from build123d import *

# Parameters (mm, degrees)
F0_W     = 14.1024803743
F0_H     = 7.6268524863
F1_DEPTH = 1
F2_W     = 9.7692511044
F2_H     = 7.6268524863
F3_DEPTH = 12.8
F5_DEPTH = 7.65
F6_R     = 2.220289971
F7_DEPTH = 5


with BuildPart() as f1:
    # F0 (on Front) → F1 (new body)
    with BuildSketch(Plane.XZ):
        with Locations((7.0512401871, 3.8134262431)):
            Rectangle(F0_W, F0_H)
    extrude(amount=F1_DEPTH)

    # F2 (on face) → F3 (join)
    with BuildSketch(Plane(origin=(0, 0, 0), x_dir=(-1, 0, 0), z_dir=(0, 1, 0))):
        with Locations((-6.9386514369, 3.8134262431)):
            Rectangle(F2_W, F2_H)
    extrude(amount=F3_DEPTH)

    # F4 (on face) → F5 (join)
    with BuildSketch(Plane.XY.offset(7.6268524863)):
        Polygon((11.8232769892, 0), (14.1024803743, 0), (11.8232769892, 12.8), align=None)
        Polygon((2.0540258847, 0), (2.0540258847, 12.8), (0, 0), align=None)
    extrude(amount=-F5_DEPTH)

    # F6 (on face) → F7 (join)
    with BuildSketch(Plane(origin=(0, 12.8, 0), x_dir=(-1, 0, 0), z_dir=(0, 1, 0))):
        with Locations((-6.9386514369, 3.8134262431)):
            Circle(F6_R)
    extrude(amount=F7_DEPTH)


solid = f1.part
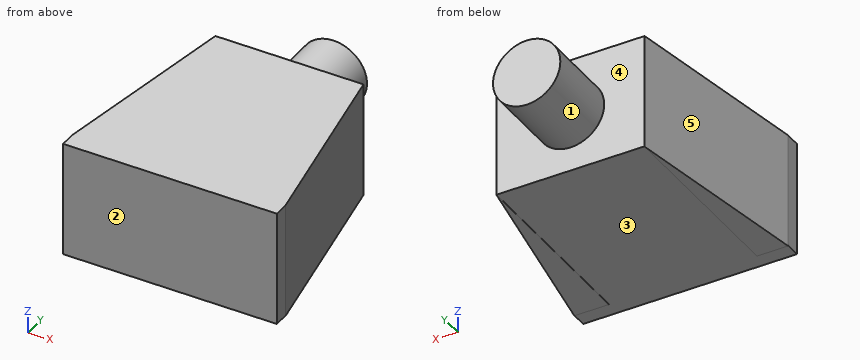
Model file for the job. Use its own axes, mm. Face numbers are marked on the shaded views. A direction names the side the tool comes from. Give positions to 0.01 mm unless a question says otherwise; leave off trailing zeros. Order: outer loops, then holes, each group sorted by start corner. A loop starts at its lowest first (then second) coordinate and runs counter-clockwise, first axis right, second up. Notation, with made-up numbers: M -19.75,-13.5 L 6.25,-13.5 A30 cw 6.25,23.5 Z; hole C 29.25,-27.5 d7. An arc over 180 degrees is marked long. Put each result on its own line as item: value. Start each with the question number.
(1) Pull direction X, two halves, no side cores. Call the marked faces 1, 2 and 3: released by +X, released by -X, zero draft, split by the parting line, or undercut.
(2) Drill centre lines: L1, parallel to Y at x = 2.25, z = 2.75; L2, parallel to Z at x = 9.5, y = 1; L3, parallel to X at y = 3.75, z = 4. Where is each one in solid material? Low to high. Write a range as [from, to].
(3) Pin check, flat tips, straight feed: pin 1 Ø7 at (x, y) = (9, 6) entering from -Z; pin 2 Ø3 at (y, z) = (2, 3.5) entering from +X; pin 3 Ø3 at (y, z) = (10.5, 5) entering from -X; pin 4 Ø1 at (y, z) = (3.5, 1) entering from -X. Stop position of each tip, or through.
(4) Band-saw the part on D-D on z = 5. Give the cut face in (x, y), then the cut area to 3 significant figures.
(5) Band-saw the part on A-A on z = 6.5. Give the cut face in (x, y), then the cut area to 3 significant figures.
(6) Band-saw the part on B-B on x = 6. Give the cut face in (y, z).
(7) Tool access for the marked faces 4 and 5: list every direction of +Z, -Z, +X, -X, +Y, -Y with a clear straight run to the whole face (end or side of a thin tool).
Results below:
1. face 1: split by the parting line
1. face 2: zero draft
1. face 3: undercut
2. L1: y = [-1, 12.8]
2. L2: z = [0, 7.63]
2. L3: x = [0.6, 13.43]
3. pin 1: stops at z = -0.02
3. pin 2: stops at x = 14.01
3. pin 3: stops at x = 1.44
3. pin 4: stops at x = 0.48
4. outline: M 0,-1 L 14.1,-1 L 14.1,0 L 11.82,12.8 L 8.82,12.8 L 8.82,17.8 L 5.06,17.8 L 5.06,12.8 L 2.05,12.8 L 0,0 Z
4. area: 186 mm2
5. outline: M 0,-1 L 14.1,-1 L 14.1,0 L 11.82,12.8 L 2.05,12.8 L 0,0 Z
5. area: 167 mm2
6. outline: M -1,0 L 12.8,0 L 12.8,1.8 L 17.8,1.8 L 17.8,5.83 L 12.8,5.83 L 12.8,7.63 L -1,7.63 Z
7. face 4: +Y
7. face 5: +Z, -Z, -X, +Y
